Check sheet for the modelled part. Datum: model origin and axes. Units: mm. A direction names the side the tool comes from. Round coordinates to 2 decimals unless told otherwise and drop trailing zeros. Order: outer loops, then holes, each group sorted by start corner. A loop starts at its lowest first (then second) coordinate and runs counter-clockwise, first axis right, second up.
Q1. Cross-section at B-B on y = 5.8. Record the cut outline in (x, z).
Q2. Cross-section at C-C on x = -3.25. Record the cut outline in (y, z).
Q3. Depth check by flat-ended pin: P1, Ø3, axis at x = 0.5, y = -3, coming from the -Z side; P2, Ø0.8, axis at x = 0, z = -1, coming from the +Y side; P3, Ø1.3, axis at x = -1.5, y = 0, coming from the +Z side. Enter the tip coordinate at first touch or a pass-through.
Q4. Cross-section at D-D on z = 46.5. Record the cut outline in (x, y), then the cut area to 3 significant figures.
Q5. Set-up check for faces 1 (the flat face through (0, 6, 0)), 2 (the flat face through (0, -0.75, -1)), 3 (the flat face through (-1, -0.8, 33)): record each of +Z, -Z, +X, -X, +Y, -Y from which the full face is reachable in a straight line by a thin tool's end or side.
Q6. Cross-section at A-A on z = 4. Record the cut outline in (x, y).
Q7. Mould release check, pull along Y, two halves, no side actions. Record for faces 4 (the flat face through (0, -6, 0)), 5 (the flat face through (-1, 0.8, 33)), 6 (the flat face through (0, 10.8, 25)): +Y half, -Y half, draft (parallel to the pull), parting line (faces both ways), or undercut.
Q8. Scan lines: probe 1 along Y at (x, z) = (1.75, 4); probe 2 along Y at (x, z) = (0.5, 44); probe 3 along Y at (x, z) = (1.75, 2). Record each from-to range of solid material in increasing order.
Autodesk Inventor part; units mm, degrees
ref_plane "YZ Plane" through (0, 0, 0) normal (1, 0, 0) x (0, 1, 0)
ref_plane "XZ Plane" through (0, 0, 0) normal (0, 1, 0) x (-1, 0, 0)
ref_plane "XY Plane" through (0, 0, 0) normal (0, 0, 1) x (1, 0, 0)
sketch "Skizze1" plane through (0, 0, 0) normal (0, 0, 1) x (1, 0, 0)
  line L0 (-5, -10.8) -> (5, -10.8)
  line L1 (5, -10.8) -> (5, 10.8)
  line L2 (5, 10.8) -> (-5, 10.8)
  line L3 (-5, 10.8) -> (-5, -10.8)
  line L4 (-5, -10.8) -> (5, 10.8) construction
  line L5 (5, -10.8) -> (-5, 10.8) construction
  point P0 (0, 0)
  dimension "d0" = 10
  dimension "d1" = 21.6
extrude "Extrusion1" add sketch "Skizze1" along normal blind 50
sketch "Skizze2" plane through (0, 0, 50) normal (0, 0, 1) x (1, 0, 0)
  line L0 (-5, 10.8) -> (-5, -10.8)
  line L1 (-5, 0.8) -> (3, 0.8)
  line L2 (3, 0.8) -> (3, -0.8)
  line L3 (3, -0.8) -> (-5, -0.8)
  line L4 (-5, -0.8) -> (-5, 0.8)
  line L5 (5, -10.8) -> (5, 10.8)
  point P0 (0, 0)
  dimension "d4" = 1.6
  dimension "d5" = 0.8
  dimension "d7" = 2
extrude "Extrusion2" cut sketch "Skizze2" against normal blind 36
sketch "Skizze3" plane through (5, -10.8, 0) normal (1, 0, 0) x (0, 0, -1)
  point P0 (0, 10.8)
sketch "Skizze4" plane through (-5, 10.8, 0) normal (-1, 0, 0) x (0, 0, 1)
  line L0 (0, 0) -> (0, -21.6)
  line L1 (0, 0) -> (0, -21.6)
  line L2 (0, -21.6) -> (50, -21.6)
  line L3 (0, 0) -> (50, 0)
  circle A0 centre (4, -5) radius 2.6
  circle A1 centre (4, -16.6) radius 2.6
  point P0 (0, -10.8)
  point P1 (0, -10)
  point P2 (0, -11.6)
  dimension "d10" = 4
  dimension "d11" = 4
  dimension "d12" = 5
  dimension "d13" = 5
  dimension "d14" = 5.2
  dimension "d15" = 5.2
extrude "Extrusion3" cut sketch "Skizze4" against normal blind 35
sketch "Skizze5" plane through (0, 0, 0) normal (0, 0, -1) x (-1, 0, 0)
  line L0 (-5, -0.75) -> (5, -0.75)
  line L1 (5, -0.75) -> (5, 0.75)
  line L2 (5, 0.75) -> (-5, 0.75)
  line L3 (-5, 0.75) -> (-5, -0.75)
  line L4 (-5, -10.8) -> (-5, 10.8)
  point P0 (0, 0)
  point P1 (-5, 0)
  dimension "d18" = 1.5
  dimension "d19" = 10
  dimension "d20" = 0
  dimension "d21" = 0.75
extrude "Extrusion4" add sketch "Skizze5" along normal blind 2.5
sketch "Skizze7" plane through (-5, 0.8, 50) normal (0, -1, 0) x (1, 0, 0)
  line L0 (0, -36) -> (0, 0)
  line L1 (10, -50) -> (0, -50)
  line L2 (0, -50) -> (0, -33.9849)
  line L3 (0, -33.9849) -> (10, -33.9849)
  line L4 (10, -33.9849) -> (10, -50)
  point P0 (5, -50)
  point P1 (0, -35)
extrude "Extrusion5" add sketch "Skizze7" along normal blind 2.5
sketch "Skizze8" plane through (-5, 0.8, 16.0151) normal (0, 0, 1) x (1, 0, 0)
  line L0 (0, 0) -> (8, 0)
  line L1 (8, -1.6) -> (0, -1.6)
  line L2 (8, 0) -> (0, 0)
  line L3 (0, 0) -> (0, -1.6)
  line L4 (0, -1.6) -> (8, -1.6)
  line L5 (8, -1.6) -> (8, 0)
  point P0 (5, -0.8)
extrude "Extrusion6" cut sketch "Skizze8" against normal blind 1.016
properties part number "Objektträgerhalterung PHM Projekt Gegenstück"
Results found:
1. outline: (-5, 0) - (5, 0) - (5, 1.4) - (-5, 1.4) - close; (-5, 6.6) - (5, 6.6) - (5, 50) - (-5, 50) - close
2. outline: (-10.8, 0) - (-0.75, 0) - (-0.75, -2.5) - (0.75, -2.5) - (0.75, 0) - (10.8, 0) - (10.8, 50) - (0.8, 50) - (0.8, 15) - (-0.8, 15) - (-0.8, 50) - (-10.8, 50) - close; hole circle Ø5.2 at (-5.8, 4); hole circle Ø5.2 at (5.8, 4)
3. P1: stops at z = 0
3. P2: stops at y = 0.75
3. P3: stops at z = 15
4. outline: (-5, -10.8) - (5, -10.8) - (5, 10.8) - (-5, 10.8) - (-5, 0.8) - (3, 0.8) - (3, -0.8) - (-5, -0.8) - close
4. area: 203 mm2
5. face 1: -Z, +X, -X, +Y
5. face 2: -Z, +X, -X, -Y
5. face 3: +Z, -X
6. outline: (-5, -10.8) - (5, -10.8) - (5, -8.4) - (-5, -8.4) - close; (-5, -3.2) - (5, -3.2) - (5, 3.2) - (-5, 3.2) - close; (-5, 8.4) - (5, 8.4) - (5, 10.8) - (-5, 10.8) - close
7. face 4: draft
7. face 5: undercut
7. face 6: +Y half
8. probe 1: y = -10.8 to -8.4, -3.2 to 3.2, 8.4 to 10.8
8. probe 2: y = -10.8 to -0.8, 0.8 to 10.8
8. probe 3: y = -10.8 to -7.46, -4.14 to 4.14, 7.46 to 10.8
